Geometry check sheet. Reference: the model listing, model coordinates, mm. A direction names the side the tool comes from. Give positions to 0.01 mm unless a question says otherwise; leave off trailing zeros. Loops run counter-clockwise (first coordinate to the right, second up) from the corner with the lowest first, then second, coordinate; pieces in that order, holes last. Notation, with made-up numbers: (48.25, 60) - (101.25, 60) arc R28 cw to (101.25, 83) - close; hole circle Ø3 at (29, -4). An arc over 180 degrees is marked (long way). One line per question, with ' | ' between items. Start each with the question number.
Autodesk Inventor part; units mm, degrees
ref_plane "YZ Plane" through (0, 0, 0) normal (1, 0, 0) x (0, 1, 0)
ref_plane "XZ Plane" through (0, 0, 0) normal (0, 1, 0) x (-1, 0, 0)
ref_plane "XY Plane" through (0, 0, 0) normal (0, 0, 1) x (1, 0, 0)
sketch "Szkic1" plane through (0, 0, 0) normal (0, 1, 0) x (-1, 0, 0)
  line L0 (-115, -5) -> (115, -5)
  line L1 (115, -5) -> (115, 5)
  line L2 (115, 5) -> (-115, 5)
  line L3 (-115, 5) -> (-115, -5)
  line L4 (-53.1699, -102.0929) -> (61.8301, 97.0929)
  line L5 (53.1699, 102.0929) -> (-61.8301, -97.0929)
  line L6 (-61.8301, -97.0929) -> (-53.1699, -102.0929)
  line L7 (61.8301, 97.0929) -> (53.1699, 102.0929)
  line L8 (61.8301, -97.0929) -> (-53.1699, 102.0929)
  line L9 (-61.8301, 97.0929) -> (53.1699, -102.0929)
  line L10 (53.1699, -102.0929) -> (61.8301, -97.0929)
  line L11 (-53.1699, 102.0929) -> (-61.8301, 97.0929)
  line L12 (115, 5) -> (-115, 5)
  line L13 (-115, -5) -> (115, -5)
  line L14 (115, -5) -> (115, 5)
  line L15 (-115, 5) -> (-115, -5)
  line L16 (53.1699, 102.0929) -> (-61.8301, -97.0929)
  line L17 (-53.1699, -102.0929) -> (61.8301, 97.0929)
  line L18 (61.8301, 97.0929) -> (53.1699, 102.0929)
  line L19 (-61.8301, -97.0929) -> (-53.1699, -102.0929)
  line L20 (-61.8301, 97.0929) -> (53.1699, -102.0929)
  line L21 (61.8301, -97.0929) -> (-53.1699, 102.0929)
  line L22 (-53.1699, 102.0929) -> (-61.8301, 97.0929)
  line L23 (53.1699, -102.0929) -> (61.8301, -97.0929)
  point P0 (0, 0)
  dimension "d6" = 10
  dimension "d7" = 5
  dimension "d8" = 230
  dimension "d9" = 115
  dimension "d12" = 360
extrude "Wyciągnięcie proste2" add sketch "Szkic1" along normal blind 3
sketch "Szkic2" plane through (0, 0, 0) normal (0, -1, 0) x (1, 0, 0)
  line L0 (-53.1699, 102.0929) -> (0, 10)
  line L1 (-61.8301, 97.0929) -> (-53.1699, 102.0929)
  point P0 (0, 0)
  point P1 (-45, 77.9423)
  point P2 (-45, -77.9423)
  point P3 (90, 0)
  dimension "d48" = 360
fillet "Zaokrąglenie3" radius 6 6 edges at (8.6603, 1.5, 5) (0, 1.5, 10) (-8.6603, 1.5, 5) (-8.6603, 1.5, -5) (0, 1.5, -10) (8.6603, 1.5, -5)
fillet "Zaokrąglenie4" radius 5 2 edges at (-53.1699, 1.5, 102.0929) (-61.8301, 1.5, 97.0929)
sketch "Szkic3" plane through (0, 0, 0) normal (0, -1, 0) x (1, 0, 0)
  point P0 (0, 0)
  point P1 (0, 0)
pattern_circular "Szyk kołowy1" count 6 over 360 about axis through (0, 0, 0) along (0, -1, 0) of "Zaokrąglenie4"
hole "Otwór1" at (-45, 0, 77.9423) at (-45, 0, -77.9423) at (90, 0, 0) direction (0, 1, 0) diameter 4.5 end through all
sketch "Szkic4" plane through (0, 0, 0) normal (0, -1, 0) x (1, 0, 0)
  circle A0 centre (0, 0) radius 106.9
  line L0 (0, 0) -> (-125.8998, 0)
  point P0 (-106.9, 0)
  point P1 (53.45, -92.5781)
  point P2 (53.45, 92.5781)
  dimension "d57" = 213.8
  dimension "d60" = 360
hole "Otwór2" at (-106.9, 0, 0) at (53.45, 0, -92.5781) at (53.45, 0, 92.5781) direction (0, 1, 0) diameter 3.242 end through all
chamfer "Faza1" distance 0.4 angle 45 6 edges at (53.45, 0, -90.9571) (90, 0, 2.25) (-45, 0, -75.6923) (-106.9, 0, 1.621) (-45, 0, 80.1923) (53.45, 0, 94.1991)
properties part number "SpiderPrimaryMirror" material "Aluminium 6061"
(1) Mould release check, pull along X, two halves, no side actions. Record for faces 1 (the face through (27.615, 1.479, 57.83)), 2 (the face through (1, 3, 0)), 3 (the face through (-114, 2, 3)): pulls with the +X half, pulls with the -X half, needs draft (parallel to the pull), parting line crosses it, or undercut.
(2) Tool access check on faces 4 (the face through (-28.25, 1.48, 58.93)), 5 (the face through (-36.275, 1.479, 52.83)), 6 (the face through (36.275, 1.479, -52.83)). Record the directions out of +Z, -Z, +X, -X, +Y, -Y that give a thin tool (end or side, any length) a straight path to the whole face; none if there is none.
(3) Section check C-C, the plane x = 84.5. Record the boundary of the cut face in (y, z), and give its area (3 significant figures).
(4) Section check B-B, the plane y = 1. Count the separate pieces of the cut face and the enclosed holes in it, and give its area (3 significant figures).
(5) Material ranges on line 1 (X direction, y = 1.05, z = 0); line 2 (Z direction, x = -14.5, y = 1.55); line 3 (Z direction, x = 52.5, y = 2), recorded low to high.
(6) Depth check by flat-ended pin: pin 1 Ø1.5 at (x, y) = (36, 1.5) entering from +Z; pin 2 Ø3.5 at (x, z) = (-45, 77.94) entering from +Y; pin 3 Ø1 at (y, z) = (0.5, 30.5) entering from +X; pin 4 Ø1.5 at (x, y) = (64, 1.5) entering from +Z. Enter the tip coordinate at first touch or a pass-through.
(7) Section check D-D, the plane z = 9. Record the boundary of the cut face in (x, y).
(8) Section check A-A, the plane z = -83.5. Record the boundary of the cut face in (x, y).
Numbers:
1) face 1: undercut | face 2: needs draft | face 3: pulls with the -X half
2) face 4: +Z, +Y, -Y | face 5: -X, +Y, -Y | face 6: +X, +Y, -Y
3) outline: (0, -5) - (3, -5) - (3, 5) - (0, 5) - close | area: 30.0 mm^2
4) separate pieces: 1 | enclosed holes: 6 | area: 6,650 mm^2
5) line 1: -115 to -108.52, -105.28 to 87.75, 92.25 to 115 | line 2: -35.11 to -15.11, -7.09 to 7.09, 15.11 to 35.11 | line 3: -99.59 to -93.89, -91.26 to -80.93, -5 to 5, 80.93 to 91.26, 93.89 to 99.59
6) pin 1: z = 73.65 | pin 2: through | pin 3: x = 23.67 | pin 4: z = 5
7) outline: (-13.4, 0) - (13.4, 0) - (13.4, 3) - (-13.4, 3) - close
8) outline: (-53.98, 0) - (-42.44, 0) - (-42.44, 3) - (-53.98, 3) - close; (42.44, 0) - (53.98, 0) - (53.98, 3) - (42.44, 3) - close
